from build123d import *

# Parameters (mm, degrees)
F1_DEPTH = 25.4


with BuildPart() as f1:
    # F0 (on Top) → F1 (new body)
    with BuildSketch(Plane.XY):
        with BuildLine():
            Line((38.1, -38.1), (38.1, 38.1))
            Line((38.1, 38.1), (16.764, 38.1))
            Line((16.764, 38.1), (16.764, 0))
            ThreePointArc((16.764, 0), (0, -16.764), (-16.764, 0))
            Line((-16.764, 0), (-16.764, 38.1))
            Line((-16.764, 38.1), (-38.1, 38.1))
            Line((-38.1, 38.1), (-38.1, -38.1))
            Line((-38.1, -38.1), (38.1, -38.1))
        make_face()
        Polygon((-54.2925, -38.1), (-38.1, -38.1), (-38.1, 38.1), (-82.55, 38.1), (-82.55, -38.1), (-66.3575, -38.1), (-66.3575, 12.7), (-60.325, 12.7), (-54.2925, 12.7), align=None)
    extrude(amount=F1_DEPTH)


solid = f1.part
Could you check a few things on this model? Use its own coordinates, in mm. A direction names the side the tool comes from. Give positions to 0.01 mm unless a question says otherwise; leave off trailing zeros. Order: outer loops, then holes, each group sorted by start corner. A loop starts at its lowest first (then second) coordinate and runs counter-clockwise, first axis right, second up.
Item 1: If we section it at B-B, the plane z = 15: Write out the boundary of the cut face in (x, y).
Item 2: For faces 1 (the face through (28, 38.1, 13)), 2 (the face through (16.764, 19, 13)), 3 (the face through (-60, 12.7, 13)), which set-ups out of +Z, -Z, +X, -X, +Y, -Y let a thin tool reach every point of the face, with its end or its side?
Item 3: I need wall thicknesses on line 1 (X direction, y = 1.5, z = 10.5); line 2 (X direction, y = 22.5, z = 19); line 3 (X direction, y = -9, z = 5.25). Which ranges of each line are inside material? Lowest first, please.
Item 4: If we section it at A-A, the plane y = 31.5: Write out the boundary of the cut face in (x, z), plus the area to 3 significant figures.
Item 5: If we section it at D-D, the plane x = 0: Write out the boundary of the cut face in (y, z), plus the area to 3 significant figures.
Item 6: If we mould it in two halves opening along X, with no side actions, what happens to faces 4 (the face through (-82.55, 1, 13)), 5 (the face through (0.37, -16.76, 12.52)), 6 (the face through (-75, -38.1, 13)), 7 (the face through (-16.764, 19, 13))? For each: pulls with the +X half, pulls with the -X half, needs draft (parallel to the pull), parting line crosses it, or undercut.
Item 7: If we section it at C-C, the plane y = -12: Write out the boundary of the cut face in (x, z), plus the area to 3 significant figures.
Values:
1. outline: (-82.55, -38.1) - (-66.36, -38.1) - (-66.36, 12.7) - (-54.29, 12.7) - (-54.29, -38.1) - (38.1, -38.1) - (38.1, 38.1) - (16.76, 38.1) - (16.76, 0) arc R16.76 cw to (-16.76, 0) - (-16.76, 38.1) - (-82.55, 38.1) - close
2. face 1: +Z, -Z, +X, -X, +Y
2. face 2: +Z, -Z, +Y
2. face 3: +Z, -Z, -Y
3. line 1: x = -82.55 to -66.36, -54.29 to -16.76, 16.76 to 38.1
3. line 2: x = -82.55 to -16.76, 16.76 to 38.1
3. line 3: x = -82.55 to -66.36, -54.29 to -14.14, 14.14 to 38.1
4. outline: (-82.55, 0) - (-16.76, 0) - (-16.76, 25.4) - (-82.55, 25.4) - close; (16.76, 0) - (38.1, 0) - (38.1, 25.4) - (16.76, 25.4) - close
4. area: 2,210 mm2
5. outline: (-38.1, 0) - (-16.76, 0) - (-16.76, 25.4) - (-38.1, 25.4) - close
5. area: 542 mm2
6. face 4: pulls with the -X half
6. face 5: undercut
6. face 6: needs draft
6. face 7: undercut
7. outline: (-82.55, 0) - (-66.36, 0) - (-66.36, 25.4) - (-82.55, 25.4) - close; (-54.29, 0) - (-11.71, 0) - (-11.71, 25.4) - (-54.29, 25.4) - close; (11.71, 0) - (38.1, 0) - (38.1, 25.4) - (11.71, 25.4) - close
7. area: 2,160 mm2
